```python
from build123d import *

# Parameters (mm, degrees)
SKETCH2_W           = 1647.9
SKETCH2_H           = 284.681734848
SKETCH2_W_2         = 36
SKETCH2_H_2         = 85.677465121
BOSS_EXTRUDE1_DEPTH = 12.7
SKETCH3_W           = 19.05
SKETCH3_H           = 284.681734848
CUT_EXTRUDE1_DEPTH  = 13.7
SKETCH4_W           = 36
SKETCH4_H           = 50.330449982
SKETCH4_H_2         = 35.349550018
CUT_EXTRUDE2_DEPTH  = 13.7


with BuildPart() as part:
    # Sketch2 → Boss-Extrude1 (new body)
    with BuildSketch(Plane.XY):
        with Locations((842.999943303, 176.189566708)):
            Rectangle(SKETCH2_W, SKETCH2_H)
        with Locations((1571.01994314, 211.688120447)):
            Rectangle(SKETCH2_W_2, SKETCH2_H_2, mode=Mode.SUBTRACT)
        with Locations((1480.459247559, 199.688120447)):
            Rectangle(SKETCH2_W_2, SKETCH2_H_2, mode=Mode.SUBTRACT)
        with Locations((1435.229386921, 193.688120447)):
            Rectangle(SKETCH2_W_2, SKETCH2_H_2, mode=Mode.SUBTRACT)
        with Locations((1390.000695887, 187.688120447)):
            Rectangle(SKETCH2_W_2, SKETCH2_H_2, mode=Mode.SUBTRACT)
        with Locations((1344.768303255, 181.688120447)):
            Rectangle(SKETCH2_W_2, SKETCH2_H_2, mode=Mode.SUBTRACT)
        with Locations((1299.538396377, 175.688120447)):
            Rectangle(SKETCH2_W_2, SKETCH2_H_2, mode=Mode.SUBTRACT)
        with Locations((1254.306140471, 169.688120446)):
            Rectangle(SKETCH2_W_2, SKETCH2_H_2, mode=Mode.SUBTRACT)
        with Locations((1209.07770281, 164.688120446)):
            Rectangle(SKETCH2_W_2, SKETCH2_H_2, mode=Mode.SUBTRACT)
        with Locations((1118.618578512, 154.688120446)):
            Rectangle(SKETCH2_W_2, SKETCH2_H_2, mode=Mode.SUBTRACT)
        with Locations((1073.383844827, 149.688120446)):
            Rectangle(SKETCH2_W_2, SKETCH2_H_2, mode=Mode.SUBTRACT)
        with Locations((1028.155686863, 146.688120446)):
            Rectangle(SKETCH2_W_2, SKETCH2_H_2, mode=Mode.SUBTRACT)
        with Locations((982.9239215, 143.688120446)):
            Rectangle(SKETCH2_W_2, SKETCH2_H_2, mode=Mode.SUBTRACT)
        with Locations((937.694704034, 142.188120446)):
            Rectangle(SKETCH2_W_2, SKETCH2_H_2, mode=Mode.SUBTRACT)
        with Locations((847.230489128, 140.688120446)):
            Rectangle(SKETCH2_W_2, SKETCH2_H_2, mode=Mode.SUBTRACT)
        with Locations((801.999943303, 140.688120446)):
            Rectangle(SKETCH2_W_2, SKETCH2_H_2, mode=Mode.SUBTRACT)
        with Locations((756.774236257, 140.688120446)):
            Rectangle(SKETCH2_W_2, SKETCH2_H_2, mode=Mode.SUBTRACT)
        with Locations((711.541406556, 140.688120446)):
            Rectangle(SKETCH2_W_2, SKETCH2_H_2, mode=Mode.SUBTRACT)
        with Locations((666.310021351, 142.188120446)):
            Rectangle(SKETCH2_W_2, SKETCH2_H_2, mode=Mode.SUBTRACT)
        with Locations((621.080803885, 143.688120446)):
            Rectangle(SKETCH2_W_2, SKETCH2_H_2, mode=Mode.SUBTRACT)
        with Locations((575.849038522, 146.688120446)):
            Rectangle(SKETCH2_W_2, SKETCH2_H_2, mode=Mode.SUBTRACT)
        with Locations((485.386146872, 154.688120446)):
            Rectangle(SKETCH2_W_2, SKETCH2_H_2, mode=Mode.SUBTRACT)
        with Locations((304.466329007, 175.688120447)):
            Rectangle(SKETCH2_W_2, SKETCH2_H_2, mode=Mode.SUBTRACT)
        with Locations((440.15644292, 159.688120446)):
            Rectangle(SKETCH2_W_2, SKETCH2_H_2, mode=Mode.SUBTRACT)
        with Locations((394.927022575, 164.688120446)):
            Rectangle(SKETCH2_W_2, SKETCH2_H_2, mode=Mode.SUBTRACT)
        with Locations((349.698584914, 169.688120446)):
            Rectangle(SKETCH2_W_2, SKETCH2_H_2, mode=Mode.SUBTRACT)
        with Locations((168.775338464, 193.688120447)):
            Rectangle(SKETCH2_W_2, SKETCH2_H_2, mode=Mode.SUBTRACT)
    extrude(amount=BOSS_EXTRUDE1_DEPTH)

    # Sketch3 → Cut-Extrude1 (cut, through all)
    with BuildSketch(Plane.XY.offset(12.7)):
        with Locations((1657.424943303, 176.189566708)):
            Rectangle(SKETCH3_W, SKETCH3_H)
        with Locations((28.574943303, 176.189566708)):
            Rectangle(SKETCH3_W, SKETCH3_H)
    extrude(amount=-CUT_EXTRUDE1_DEPTH, mode=Mode.SUBTRACT)

    # Sketch4 → Cut-Extrude2 (cut, through all)
    with BuildSketch(Plane.XY.offset(12.7)):
        with Locations((123.545338464, 218.853345438)):
            Rectangle(SKETCH4_W, SKETCH4_H)
        with Locations((123.545338464, 176.013345438)):
            Rectangle(SKETCH4_W, SKETCH4_H_2)
    extrude(amount=-CUT_EXTRUDE2_DEPTH, mode=Mode.SUBTRACT)


solid = part.part
```
Model file for the job. Use its own axes, mm. Round coordinates to 2 decimals unless told otherwise and drop trailing zeros. Loops run counter-clockwise (first coordinate to the right, second up) from the corner with the lowest first, then second, coordinate; pieces in that order, holes last. Notation, with made-up numbers: M 7.25,-27.75 L 64.25,-27.75 A30 ccw 64.25,3.25 Z; hole C 12.25,71 d4. An arc over 180 degrees is marked long. Put each result on its own line as item: value. Start each with the question number.
Item 1: Cut at A-A (x = 933.5). List the corners of the cut face in (y, z).
Item 2: Cut at B-B (z = 10.5). Give the number of separate pieces and of enclosed holes in the cut face, then the cut area to 3 significant figures.
Item 3: Drill centre lines: line 1 along Y through (x, z) = (1037, 2.5); line 2 along X through (y, z) = (237, 7); line 3 along Y through (x, z) = (1477, 10.25). Where is each one in solid material? Low to high.
Answer block:
1. outline: M 33.85,0 L 99.35,0 L 99.35,12.7 L 33.85,12.7 Z; M 185.03,0 L 318.53,0 L 318.53,12.7 L 185.03,12.7 Z
2. separate pieces: 1
2. enclosed holes: 27
2. area: 375,000 mm2
3. line 1: 33.85 to 103.85, 189.53 to 318.53
3. line 2: 38.1 to 105.55, 141.55 to 1462.46, 1498.46 to 1553.02, 1589.02 to 1647.9
3. line 3: 33.85 to 156.85, 242.53 to 318.53
